CAD build for the part. Positions are in the model's coordinates, mm. Coordinates: 2 decimals unless noted, no trailing zeros. Loops run counter-clockwise (first coordinate to the right, second up) from the corner with the lowest first, then second, coordinate; pieces in that order, holes last. Notation, with made-up numbers: (56.5, 80) -> (78.5, 80) arc R13 cw to (78.5, 103) -> close; hole circle Ø5 at (35.5, 53). An arc over 180 degrees is marked (long way). Write item = value, one per line. Start each with the question number.
(1) Band-saw the part on B-B (z = 1.5). Write the cut outline in (x, y) (3 decimals).
(2) Band-saw the part on A-A (y = 0). Write the cut outline in (x, z) (3 decimals).
(3) Pull direction Y, two halves, no side cores. Call faces 1 (the face through (-14.996, -0.33, 1.493)), 2 (the face through (26, 0, 3)), 3 (the face through (48.476, 0.067, 1.479)), 4 (the face through (4.91, 1.55, 1.52)): +Y half, -Y half, draft (parallel to the pull), parting line (faces both ways), or undercut.
(4) Drill centre lines: line 1 (Y direction, x = 50, z = 1.9) (3 decimals); line 2 (X direction, y = 0.5, z = 2.6); line 3 (Y direction, x = 0, z = 2.15). Where is each one in solid material? Low to high. Write a range as from..to.
```python
from build123d import *

# Parameters (mm, degrees)
EXTRUDE_1_DEPTH     = 3
SKETCH_1_3_R        = 1.525
CUT_EXTRUDE_1_DEPTH = 5
FILLET_1_R          = 1
SKETCH_2_R          = 5.15
CUT_EXTRUDE_2_DEPTH = 5


with BuildPart() as part:
    # 草图1 → 凸台-拉伸1 (new body)
    with BuildSketch(Plane.XY):
        with BuildLine():
            Line((0, 15), (50, 15))
            ThreePointArc((50, 15), (65, 0), (50, -15))
            Line((50, -15), (0, -15))
            ThreePointArc((0, -15), (-15, 0), (0, 15))
        make_face()
    extrude(amount=EXTRUDE_1_DEPTH)

    # 草图1<3> → 切除-拉伸1 (cut)
    with BuildSketch(Plane.XY):
        with Locations((50, 0)):
            Circle(SKETCH_1_3_R)
    extrude(amount=CUT_EXTRUDE_1_DEPTH, mode=Mode.SUBTRACT)

    # 圆角1
    fillet_1_edges = [part.edges().sort_by_distance(p)[0] for p in [
        (65, 0, 3),
        (25, 15, 3),
        (-15, 0, 3),
        (25, 15, 0),
        (65, 0, 0),
        (25, -15, 0),
        (-15, 0, 0),
        (25, -15, 3),
    ]]
    fillet(fillet_1_edges, radius=FILLET_1_R)

    # 草图2 → 切除-拉伸2 (cut)
    with BuildSketch(Plane.XY.offset(3)):
        Circle(SKETCH_2_R)
    extrude(amount=-CUT_EXTRUDE_2_DEPTH, mode=Mode.SUBTRACT)


solid = part.part
```
Findings below:
q1.outline = (0, -15) -> (50, -15) arc R15 ccw to (50, 15) -> (0, 15) arc R15 ccw to start; hole circle Ø10.3 at (0, 0); hole circle Ø3.05 at (50, 0)
q2.outline = (-15, 1) arc R1 ccw to (-14, 0) -> (-5.15, 0) -> (-5.15, 3) -> (-14, 3) arc R1 ccw to (-15, 2) -> close; (5.15, 0) -> (48.475, 0) -> (48.475, 3) -> (5.15, 3) -> close; (51.525, 0) -> (64, 0) arc R1 ccw to (65, 1) -> (65, 2) arc R1 ccw to (64, 3) -> (51.525, 3) -> close
q3.face_1 = parting line
q3.face_2 = draft
q3.face_3 = undercut
q3.face_4 = undercut
q4.line_1 = -15..-1.525, 1.525..15
q4.line_2 = -14.79..-5.13, 5.13..48.56, 51.44..64.79
q4.line_3 = -14.99..-5.15, 5.15..14.99
